Geometry: final body of the model. Coordinates: model frame, mm. Face numbers are marked on the shaded views. A direction names the side the tool comes from. Give positions to 0.01 mm unless a question says otherwise; leave off trailing zeros. Write each loop counter-clockwise with the first axis right and the second up, starting at its lowest first coordinate (ties: lowest second). Pieces come first, ordered by that corner, then holes. Notation, with made-up numbers: M -8.75,40.25 L 9.25,40.25 A16 ccw 9.25,54.25 Z; hole C 75,-12.5 d2. An arc over 180 degrees is marked long. Use one line per item in the form item = value. Start each with the question number.
Item 1: Contact query for flat-ended pins moving along their axis: P1, Ø2, axis at x = -1, z = 0, coming from the +Y side; P2, Ø1.2, axis at x = 10, z = 0, coming from the -Y side. Output: stop coordinate, or through.
Item 2: Section query C-C on z = -4.5. Return loops of the section in (x, y), then the cut area to 3 significant figures.
Item 3: Section query A-A on y = 7. Return loops of the section in (x, z) (3 decimals).
Item 4: Material intervals for line 1 along Z through (x, y) = (10, 4.25) (3 decimals); line 2 along Z through (x, y) = (0, 3.55); line 3 along X through (y, z) = (2, -1.5), sorted ascending. Write a range as from..to.
Item 5: Pull-direction query (X, two-part tool) for the marked faces 1, 2, 3 and 4; classes: released by +X, released by -X, zero draft, split by the parting line, or undercut.
Item 6: Section query B-B on y = 2. Return loops of the section in (x, z) (3 decimals).
Item 7: Access query for the marked faces 5, 6 and 7. Directions: +Z, -Z, +X, -X, +Y, -Y. A direction counts if a zero-diameter tool reaches every point of the face in a straight line with its end or side. Return the directions, or none.
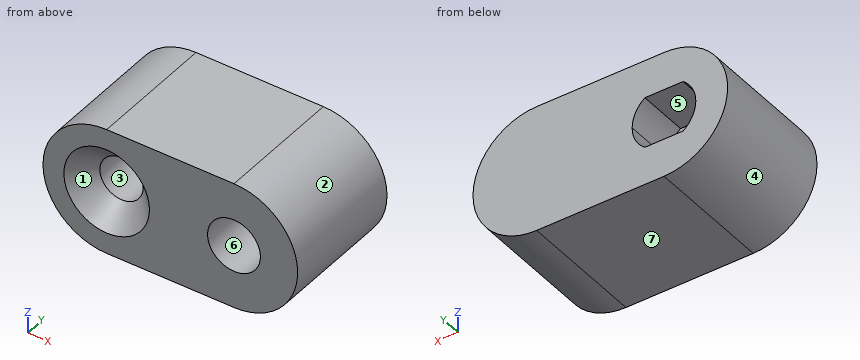
from build123d import *

# Parameters (mm, degrees)
EXTRUDE_1_DEPTH              = 10
CUT_EXTRUDE_1_DEPTH          = 4
HOLE_WIZARD_M3_1_D           = 3.4
HOLE_WIZARD_M3_1_DEPTH       = 8.1
HOLE_WIZARD_M3_1_CSINK_D     = 6.72
HOLE_WIZARD_M3_1_CSINK_ANGLE = 90
HOLE_WIZARD_M3_1_TIP         = 1.021463052
HOLE_WIZARD_1_D              = 4.15
HOLE_WIZARD_1_DEPTH          = 7.5


with BuildPart() as part:
    # 草图1 → 凸台-拉伸1 (new body)
    with BuildSketch(Plane(origin=(0, 0, 0), x_dir=(1, 0, 0), z_dir=(0, 1, 0))):
        with BuildLine():
            Line((0, 5), (10, 5))
            ThreePointArc((10, 5), (15, 0), (10, -5))
            Line((10, -5), (0, -5))
            ThreePointArc((0, -5), (-5, 0), (0, 5))
        make_face()
    extrude(amount=EXTRUDE_1_DEPTH)

    # 草图2 → 切除-拉伸1 (cut)
    with BuildSketch(Plane(origin=(0, 10, 0), x_dir=(1, 0, 0), z_dir=(0, 1, 0))):
        with BuildLine():
            Line((1.5, 2), (-1.5, 2))
            ThreePointArc((-1.5, 2), (-2.5, 0), (-1.5, -2))
            Line((-1.5, -2), (1.5, -2))
            ThreePointArc((1.5, -2), (2.236067977, -1.118033989), (2.5, 0))
            ThreePointArc((2.5, 0), (2.236067977, 1.118033989), (1.5, 2))
        make_face()
    extrude(amount=-CUT_EXTRUDE_1_DEPTH, mode=Mode.SUBTRACT)

    # M3 六角凹锥坑螺钉的锥形沉头孔1
    with Locations(Plane(origin=(0, 0, 0), x_dir=(-1, 0, 0), z_dir=(0, -1, 0))):
        with Locations((0, 0)):
            CounterSinkHole(HOLE_WIZARD_M3_1_D / 2, HOLE_WIZARD_M3_1_CSINK_D / 2, depth=HOLE_WIZARD_M3_1_DEPTH, counter_sink_angle=HOLE_WIZARD_M3_1_CSINK_ANGLE)
            with Locations((0, 0, -(HOLE_WIZARD_M3_1_DEPTH + HOLE_WIZARD_M3_1_TIP / 2))):  # 118° drill point
                Cone(0, HOLE_WIZARD_M3_1_D / 2, HOLE_WIZARD_M3_1_TIP, mode=Mode.SUBTRACT)

    # 孔1
    with Locations(Plane(origin=(0, 0, 0), x_dir=(-1, 0, 0), z_dir=(0, -1, 0))):
        with Locations((-10, 0)):
            Hole(HOLE_WIZARD_1_D / 2, depth=HOLE_WIZARD_1_DEPTH)


solid = part.part
Answer sheet:
q1.P1 = 6
q1.P2 = 7.5
q2.outline = M -2.18,0 L 12.18,0 L 12.18,10 L -2.18,10 Z
q2.area = 144 mm2
q3.outline = M 0,-5 L 10,-5 A5 ccw 10,5 L 0,5 A5 ccw Z; hole M -1.5,-2 L 1.5,-2 A2.5 ccw 1.5,2 L -1.5,2 A2.5 ccw Z; hole C 10,0 d4.15
q4.line_1 = -5..-2.075, 2.075..5
q4.line_2 = -5..-1.7, 1.7..5
q4.line_3 = -4.77..-0.8, 0.8..8.57, 11.43..14.77
q5.face_1 = undercut
q5.face_2 = released by +X
q5.face_3 = undercut
q5.face_4 = released by -X
q6.outline = M 0,-5 L 10,-5 A5 ccw 10,5 L 0,5 A5 ccw Z; hole C 0,0 d3.4; hole C 10,0 d4.15
q7.face_5 = +Y
q7.face_6 = -Y
q7.face_7 = -Z, +X, -X, +Y, -Y
